```python
from build123d import *

# Parameters (mm, degrees)
F1_DEPTH = 3
F2_R     = 5


with BuildPart() as f1:
    # F0 (on Front) → F1 (new body)
    with BuildSketch(Plane.XZ):
        Polygon((20, 0), (0, 0), (-9.969531, -43.881755), (5.030469, -43.881755), (10, -9.236355), (21.716592, -7.555729), align=None)
        Polygon((29.969531, -43.881755), (21.716592, -7.555729), (10, -9.236355), (14.969531, -43.881755), align=None)
    extrude(amount=F1_DEPTH)

    # F2
    f2_edges = [f1.edges().sort_by_distance(p)[0] for p in [
        (-9.969531, -1.5, -43.881755),
        (5.030469, -1.5, -43.881755),
        (14.969531, -1.5, -43.881755),
        (29.969531, -1.5, -43.881755),
    ]]
    fillet(f2_edges, radius=F2_R)


solid = f1.part
```
Work out the finished part from the listing and answer in its coordinate system (mm). A direction names the side the tool comes from. Give positions to 0.01 mm unless a question says otherwise; leave off trailing zeros. Order: outer loops, then holes, each group sorted by start corner. A loop starts at its lowest first (then second) coordinate and runs counter-clockwise, first axis right, second up.
1. Section A-A, the plane z = -16.5 is taken. Determine the outline of the cut face in (x, y), and give its area (3 significant figures).
Result sheet:
outline: (-3.75, -3) - (8.96, -3) - (8.96, 0) - (-3.75, 0) - close; (11.04, -3) - (23.75, -3) - (23.75, 0) - (11.04, 0) - close
area: 76.2 mm2
2. Section B-B, the plane y = -1.6 is taken. Determine the outline of the cut face in (x, z).
Result sheet:
outline: (-8.58, -37.77) arc R5 ccw to (-3.71, -43.88) - (0.7, -43.88) arc R5 ccw to (5.65, -39.59) - (10, -9.24) - (14.35, -39.59) arc R5 ccw to (19.3, -43.88) - (23.71, -43.88) arc R5 ccw to (28.58, -37.77) - (20, 0) - (0, 0) - close
3. Straight lines are drawn through the part: L1, parallel to X at y = -2.1, z = -40; L2, parallel to X at y = -0.9, z = -24.5; L3, parallel to Z at x = 4.5, y = -2.25. For each, find the intervals that lie inside material, in ascending order.
Result sheet:
L1: x = -8.58 to 5.57, 14.43 to 28.58
L2: x = -5.57 to 7.81, 12.19 to 25.57
L3: z = -42.13 to 0
4. For faces 5 (the flat face through (-2, -1, -43.882)), 6 (the cylindrical face through (15.991, -1.521, -42.627)), determine the directions among +Z, -Z, +X, -X, +Y, -Y from which every point of the face is accessible in a straight line to the end or side of a thin tool.
Result sheet:
face 5: -Z, +X, -X, +Y, -Y
face 6: -Z, +Y, -Y
5. The mould has two halves that part along X. Classify faces 1 (the cylindrical face through (27.574, -1.521, -42.05)), 2 (the flat face through (7.79, -1.48, -24.63)), 3 (the flat face through (14, -3, -22)), 4 (the cylindrical face through (3.933, -1.521, -42.693)): released by +X, released by -X, zero draft, split by the parting line, or undercut.
Result sheet:
face 1: released by +X
face 2: undercut
face 3: zero draft
face 4: undercut
6. Section D-D, the plane z = -30 is taken. Determine the outline of the cut face in (x, y).
Result sheet:
outline: (-6.82, -3) - (7.02, -3) - (7.02, 0) - (-6.82, 0) - close; (12.98, -3) - (26.82, -3) - (26.82, 0) - (12.98, 0) - close
7. Section C-C, the plane x = 4.5 is taken. Determine the outline of the cut face in (y, z), and give its area (3 significant figures).
Result sheet:
outline: (-3, -42.13) - (0, -42.13) - (0, 0) - (-3, 0) - close
area: 126 mm2
